For this review, take the finished solid that the model builds, in its own axes (mm). A direction names the side the tool comes from. Give positions to 0.01 mm unless a question says otherwise; leave off trailing zeros. Order: outer loops, then holes, each group sorted by start corner. A loop starts at its lowest first (then second) coordinate and runs counter-clockwise, first axis right, second up. Notation, with made-up numbers: (4.25, 30.25) -> (25.25, 30.25) arc R5 cw to (25.25, 36.25) -> close; hole circle Ø2 at (5, 12). An arc over 180 degrees is marked (long way). Return JSON: item names as keys, results as strings. Group by question number.
1) To check wall thickness, follow line 1 along X through (y, z) = (44, 83.5); line 2 along Y through (x, z) = (-10.5, 14.5); line 3 along Y through (x, z) = (10, 67.5). State the ranges of each line that lie inside material, in increasing order.
2) For faces 4 (the face through (12.621, -1, 13)), 5 (the face through (-25.479, 43, 64)), 6 (the face through (-38, 36.896, 64)), 7 (the face through (-38.001, -26.782, 12.878)), list the 3-axis set-ups (+Z, -Z, +X, -X, +Y, -Y) from which the entire face can be reached by the end or side of a thin tool; tool diameter is ignored.
3) Add section C-C (x = 5.5). Give the boundary of the cut face in (y, z), then the cut area to 3 significant figures.
4) Add section B-B (z = 21.5). Give the boundary of the cut face in (x, y), then the cut area to 3 significant figures.
5) Insertion check: P1, Ø1, axis at x = -22.5, y = -29, coming from the +Z side; P2, Ø8, axis at x = 13.5, z = 47, coming from the -Y side. Each pin has a flat end and moves straight along its axis. Give the tip position at first contact, or say it passes through.
6) Add section D-D (z = 66). Give the boundary of the cut face in (x, y).
7) The part is to be moulded in two halves that separate along Y. For faces 1 (the face through (0, 11.496, 13)), 2 (the face through (38.199, -26.426, 12.878)), 3 (the face through (-1, 62.296, 50)), say which applies: released by +Y, released by -Y, zero draft, split by the parting line, or undercut.
8) Add section A-A (y = 2). Give the boundary of the cut face in (x, z), then the cut area to 3 significant figures.
from build123d import *

# Parameters (mm, degrees)
F0_W     = 101.6
F0_H     = 101.6
F1_DEPTH = 101.6
F2_W     = 101.6
F2_H     = 76.2
F3_DEPTH = 76.2
F4_W     = 50.8
F4_H     = 12.7
F5_DEPTH = 76.2
F6_W     = 25.4
F6_H     = 25.4
F7_DEPTH = 75.438
F9_DEPTH = 57.912


with BuildPart() as f1:
    # F0 (on Top) → F1 (new body)
    with BuildSketch(Plane.XY):
        with Locations((-0.078824, 11.495703)):
            Rectangle(F0_W, F0_H)
    extrude(amount=F1_DEPTH)

    # F2 (on face) → F3 (cut)
    with BuildSketch(Plane.XY.offset(101.6)):
        with Locations((-0.078824, -1.204297)):
            Rectangle(F2_W, F2_H)
    extrude(amount=-F3_DEPTH, mode=Mode.SUBTRACT)

    # F4 (on face) → F5 (cut)
    with BuildSketch(Plane.XY.offset(101.6)):
        with Locations((-0.078824, 43.245703)):
            Rectangle(F4_W, F4_H)
    extrude(amount=-F5_DEPTH, mode=Mode.SUBTRACT)

    # F6 (on face) → F7 (cut)
    with BuildSketch(Plane.XY.offset(25.4)):
        with Locations((-0.078824, -1.204297)):
            Rectangle(F6_W, F6_H)
    extrude(amount=-F7_DEPTH, mode=Mode.SUBTRACT)

    # F8 (on face) → F9 (cut)
    with BuildSketch(Plane.XY.offset(25.4)):
        Polygon((-50.878824, -13.904297), (-50.878824, -39.304297), (-25.478824, -39.304297), align=None)
        Polygon((25.321176, -39.304297), (50.721176, -39.304297), (50.721176, -13.904297), align=None)
    extrude(amount=-F9_DEPTH, mode=Mode.SUBTRACT)


solid = f1.part
Evaluation:
{
 "1": {"line 1": "-50.88 to -25.48, 25.32 to 50.72", "line 2": "-39.3 to -13.9, 11.5 to 62.3", "line 3": "49.6 to 62.3"},
 "2": {"face 4": "+Z, -Z", "face 5": "+Z, -Y", "face 6": "+Z, +X, -X, -Y", "face 7": "+Z, -Z, -X, -Y"},
 "3": {"outline": "(-39.3, 0) -> (-13.9, 0) -> (-13.9, 25.4) -> (-39.3, 25.4) -> close; (11.5, 0) -> (62.3, 0) -> (62.3, 101.6) -> (49.6, 101.6) -> (49.6, 25.4) -> (11.5, 25.4) -> close", "area": "2,900 mm^2"},
 "4": {"outline": "(-50.88, -13.9) -> (-25.48, -39.3) -> (25.32, -39.3) -> (50.72, -13.9) -> (50.72, 62.3) -> (-50.88, 62.3) -> close; hole (-12.78, -13.9) -> (12.62, -13.9) -> (12.62, 11.5) -> (-12.78, 11.5) -> close", "area": "9,030 mm^2"},
 "5": {"P1": "z = 25.4", "P2": "y = 49.6"},
 "6": {"outline": "(-50.88, 36.9) -> (-25.48, 36.9) -> (-25.48, 49.6) -> (25.32, 49.6) -> (25.32, 36.9) -> (50.72, 36.9) -> (50.72, 62.3) -> (-50.88, 62.3) -> close"},
 "7": {"face 1": "undercut", "face 2": "released by -Y", "face 3": "released by +Y"},
 "8": {"outline": "(-50.88, 0) -> (-12.78, 0) -> (-12.78, 25.4) -> (-50.88, 25.4) -> close; (12.62, 0) -> (50.72, 0) -> (50.72, 25.4) -> (12.62, 25.4) -> close", "area": "1,940 mm^2"}
}
